Build history of the part. All positions in model axes, mm. A direction names the side the tool comes from. Round coordinates to 2 decimals unless told otherwise and drop trailing zeros. Loops run counter-clockwise (first coordinate to the right, second up) from the corner with the lowest first, then second, coordinate; pieces in that order, holes last. Notation, with made-up numbers: (27.5, 89.25) -> (58.5, 89.25) arc R25 ccw to (58.5, 104.25) -> close; hole circle Ø3 at (-32.5, 87). An arc over 180 degrees is marked (long way). Put each result on its own line as item: value. Start each with the question number.
Item 1: Pull direction X, two halves, no side cores. Call faces 3 (the flat face through (-12, 3, -3)), 4 (the flat face through (-8.5, -2, -7)), 5 (the cylindrical face through (0.09, 0.69, -3.1)): +X half, -X half, draft (parallel to the pull), parting line (faces both ways), or undercut.
Item 2: Cut at C-C, the plane x = 3.75. List the corners of the cut face in (y, z) (3 decimals), plus the area to 3 significant figures.
Item 3: Drill centre lines: probe 1 along Z at (x, y) = (4.75, 0) (3 decimals); probe 2 along Z at (x, y) = (-11, 2.5); probe 3 along Y at (x, z) = (-9, 0.5). Where is each one in solid material? Low to high. Write a range as [from, to].
Item 4: Flat gauge pins, fed straight in: pin 1 Ø2 at (x, y) = (6, 3.5) entering from +Z; pin 2 Ø4 at (x, y) = (-3.5, 5) entering from -Z; pin 3 Ø2 at (x, y) = (2, 4.5) entering from +Z. Where does each tip first touch, or does it go through?
Item 5: Tool access for faces 1 (the cylindrical face through (-9.979, -7.493, 0.33)), 2 (the cylindrical face through (-7.942, 4.259, -5.555)): list every direction of +Z, -Z, +X, -X, +Y, -Y with a clear straight run to the whole face (end or side of a thin tool).
```python
from build123d import *

# Parameters (mm, degrees)
F0_R     = 7.5
F1_DEPTH = 12
F3_D     = 6.35
F4_SIZE  = 0.5
F5_W     = 1.1
F5_H     = 3.9801998064


with BuildPart() as f1:
    # F0 (on Right) → F1 (new body, symmetric)
    with BuildSketch(Plane.YZ):
        Circle(F0_R)
    extrude(amount=F1_DEPTH, both=True)

    # F3 (through all)
    with Locations(Plane.YZ.offset(12)):
        with Locations((0, 0)):
            Hole(F3_D / 2)

    # F4
    f4_edges = [f1.edges().sort_by_distance(p)[0] for p in [
        (12, -7.5, 0),
        (-12, -7.5, 0),
        (-12, -3.175, 0),
    ]]
    chamfer(f4_edges, length=F4_SIZE)

    # F5 (on Front) → F6 (revolve, cut)
    with BuildSketch(Plane.XZ):
        with Locations((-7.95, 8.9900999032)):
            Rectangle(F5_W, F5_H)
        with Locations((7.95, 8.9900999032)):
            Rectangle(F5_W, F5_H)
    revolve(axis=Axis((-0.5466132425, 0, 0), (1, 0, 0)), mode=Mode.SUBTRACT)


solid = f1.part
```
Reply:
1. face 3: -X half
1. face 4: undercut
1. face 5: draft
2. outline: circle Ø15 at (0, 0); hole circle Ø6.35 at (0, 0)
2. area: 145 mm^2
3. probe 1: z = [-7.5, -3.175], [3.175, 7.5]
3. probe 2: z = [-7.07, -1.96], [1.96, 7.07]
3. probe 3: y = [-7.48, -3.14], [3.14, 7.48]
4. pin 1: stops at z = 7.07
4. pin 2: stops at z = -6.87
4. pin 3: stops at z = 6.63
5. face 1: +X, -X
5. face 2: none
